Geometry check sheet. Reference: the model listing, model coordinates, mm. A direction names the side the tool comes from. Coordinates: 2 decimals unless noted, no trailing zeros. Loops run counter-clockwise (first coordinate to the right, second up) from the corner with the lowest first, then second, coordinate; pieces in that order, holes last.
from build123d import *

# Parameters (mm, degrees)
F1_DEPTH = 63.5
F2_DEPTH = 25.4
F0_W     = 25.4
F0_H     = 19.05
F3_DEPTH = 38.1
F6_DEPTH = 91.186
F7_R     = 12.69999


# Not quite as in the source:
# - a fillet or chamfer is up to 0.001 mm smaller than in the source, because OpenCascade refuses the exact size


with BuildPart() as f1:
    # F0 (on Front) → F1 (new body, symmetric)
    with BuildSketch(Plane.XZ):
        Polygon((22.225, 9.525), (-41.275, 9.525), (-41.275, -9.525), (41.275, -9.525), (41.275, 9.525), align=None)
    extrude(amount=F1_DEPTH, both=True)

    # F0 (on Front) → F2 (join, symmetric)
    with BuildSketch(Plane.XZ):
        with BuildLine():
            add(Edge.make_bspline(
                [(-41.275, 9.525), (-39.5856284224, 39.4828766469), (13.870125209, 59.4306981306), (53.8854342407, 61.7722898912)],
                knots=[0, 0, 0, 0, 108.5245810491, 108.5245810491, 108.5245810491, 108.5245810491], degree=3))
            Line((-41.275, 9.525), (22.225, 9.525))
            Line((22.225, 9.525), (22.225, 27.0002))
            ThreePointArc((22.225, 27.0002), (31.3258777096, 50.5133948686), (53.8854342407, 61.7722898912))
        make_face()
    extrude(amount=F2_DEPTH, both=True)

    # F0 (on Front) → F3 (join, symmetric)
    with BuildSketch(Plane.XZ):
        with BuildLine():
            Line((22.225, 27.0002), (22.225, 9.525))
            Line((22.225, 9.525), (41.275, 9.525))
            Line((41.275, 9.525), (41.275, 27.0002))
            ThreePointArc((41.275, 27.0002), (45.9246798487, 38.2255201513), (57.15, 42.8752))
            Line((57.15, 42.8752), (60.325, 42.8752))
            Line((60.325, 42.8752), (60.325, 61.9252))
            Line((60.325, 61.9252), (57.15, 61.9252))
            add(Edge.make_bspline(
                [(53.8854342407, 61.7722898912), (54.9842067368, 61.8365871986), (56.0728453275, 61.8876096574), (57.15, 61.9252)],
                knots=[108.5245810491, 108.5245810491, 108.5245810491, 108.5245810491, 111.5045361635, 111.5045361635, 111.5045361635, 111.5045361635], degree=3))
            ThreePointArc((53.8854342407, 61.7722898912), (31.3258777096, 50.5133948686), (22.225, 27.0002))
        make_face()
        with Locations((73.025, 52.4002)):
            Rectangle(F0_W, F0_H)
    extrude(amount=F3_DEPTH, both=True)

    # F0 (on Front) → F4 (revolve)
    with BuildSketch(Plane.XZ):
        Polygon((85.725, 66.675), (85.725, 61.9252), (85.725, 42.8752), (85.725, 38.1), (111.125, 38.1), (111.125, 66.675), align=None)
    revolve(axis=Axis((85.725, 0, 52.3875), (0, 0, 1)))

    # F5 (on face) → F6 (cut)
    with BuildSketch(Plane.XY.offset(66.675)):
        Polygon((101.2713760138, -8.9757043765), (101.2713760138, 8.9757043765), (85.725, 17.9514087529), (70.1786239862, 8.9757043765), (70.1786239862, -8.9757043765), (85.725, -17.9514087529), align=None)
    extrude(amount=-F6_DEPTH, mode=Mode.SUBTRACT)

    # F7 (radius 12.7 in the source; OpenCascade refuses exactly that, so slightly less here)
    f7_edges = [f1.edges().sort_by_distance(p)[0] for p in [
        (85.725, -38.1, 52.4002),
        (85.725, 38.1, 52.4002),
        (41.275, -63.5, 0),
        (-41.275, -63.5, 0),
        (41.275, 63.5, 0),
    ]]
    fillet(f7_edges, radius=F7_R)


solid = f1.part
1) Section check B-B on y = -40. Record the cut outline in (x, z) (3 decimals).
Data:
outline: (-41.275, -9.525) - (41.275, -9.525) - (41.275, 9.525) - (-41.275, 9.525) - close
2) Material ranges on probe 1 along Z at (x, y) = (27, 44.5) (3 decimals); probe 2 along X at (y, z) = (-37, 28); probe 3 along X at (y, z) = (-51.5, -2), recorded low to high.
Data:
probe 1: z = -9.525 to 9.525
probe 2: x = 22.24 to 41.31
probe 3: x = -41.26 to 41.26
3) Mould release check, pull along X, two halves, no side actions. Record for faces 5 (the flat face through (59, -1, 42.875)), 6 (the cylindrical face through (82.103, 34.281, 52.534)), 7 (the flat face through (59, -1, 61.925)): +X half, -X half, draft (parallel to the pull), parting line (faces both ways), or undercut.
Data:
face 5: undercut
face 6: +X half
face 7: draft
4) Section check A-A on x = 99. Record the cut outline in (y, z) (3 decimals), and give its area (3 significant figures).
Data:
outline: (-21.655, 38.1) - (-10.287, 38.1) - (-10.287, 66.675) - (-21.655, 66.675) - close; (10.287, 38.1) - (21.655, 38.1) - (21.655, 66.675) - (10.287, 66.675) - close
area: 650 mm2
5) Depth check by flat-ended pin: pin 1 (15 mm diameter, centred on x = 49.5, z = 33, fed in from -Y); pin 2 (4 mm diameter, centred on y = -30, z = 21.5, fed in from -X) (3 decimals); pin 3 (19.5 mm diameter, centred on y = -2, z = 47, fed in from -X); pin 4 (9 mm diameter, centred on y = -3, z = 58, fed in from +X) (3 decimals). Enter the tip coordinate at first touch or a pass-through.
Data:
pin 1: stops at y = -38.1
pin 2: stops at x = 22.225
pin 3: stops at x = -22.9
pin 4: stops at x = 111.125
6) Access from +Z, -Z, +X, -X, +Y, -Y to the whole of each face (thin tool, end or side, straight path). Record for faces 1 (the flat face through (70.179, 0, 53)), 2 (the flat face through (41.275, -1, 8)), 3 (the flat face through (-4, -25.4, 30)), 4 (the cylindrical face through (31.57, 31.66, 50.78)).
Data:
face 1: +Z, -Z
face 2: -Z, +X, +Y, -Y
face 3: +Z, -X, -Y
face 4: +Z, -X, +Y
7) Section check C-C on y = -53. Record the cut outline in (x, z) (3 decimals), and give its area (3 significant figures).
Data:
outline: (-41.083, -9.525) - (41.083, -9.525) - (41.083, 9.525) - (-41.083, 9.525) - close
area: 1,570 mm2
